Autodesk Inventor part; units mm, degrees
ref_plane "YZ Plane" through (0, 0, 0) normal (1, 0, 0) x (0, 1, 0)
ref_plane "XZ Plane" through (0, 0, 0) normal (0, 1, 0) x (-1, 0, 0)
ref_plane "XY Plane" through (0, 0, 0) normal (0, 0, 1) x (1, 0, 0)
sketch "sk_main" plane through (0, 0, 0) normal (1, 0, 0) x (0, 1, 0)
  line L0 (-8, 0) -> (30.5, 0)
  line L1 (0, -15.9) -> (0, 14.9)
  line L2 (25, -7.5) -> (0, -7.5)
  line L3 (0, -7.5) -> (0, 9)
  line L4 (25, -11.5) -> (-2.5, -11.5)
  line L5 (-2.5, -11.5) -> (-2.5, 10.5)
  line L6 (0, 10.5) -> (0, -11.5)
  line L7 (25, -7.5) -> (25, -11.5)
  line L8 (-2.5, 10.5) -> (0, 10.5)
  point P0 (0, 0)
  dimension "d5" = 2.5
  dimension "d35" = 25
  dimension "d37" = 4
  dimension "d38" = 18
  dimension "d58" = 10.5
extrude "ext_main_back" [suppressed]
extrude "ext_main_front" add sketch "sk_main" along normal mid plane 12.15 contours L5 L8 L1 L0 | L0 L1 L4 L5
sketch "sk_front" plane through (0, 0, 0) normal (0, 1, 0) x (-1, 0, 0)
  line L0 (0, -22.55) -> (0, 16.3)
  line L1 (12.1092, 0) -> (-12.1092, 0)
  circle A0 centre (0, 0) radius 3.4
  circle A1 centre (5.075, 0) radius 1
  circle A2 centre (-5.075, 0) radius 1
  circle A3 centre (0, 0) radius 8 construction
  circle A4 centre (0, -9) radius 8 construction
  circle A5 centre (0, -9) radius 1
  line L2 (8.6494, -4.5) -> (-8.6494, -4.5) construction
  line L3 (-6.075, 10.5) -> (-6.075, -11.5)
  line L4 (6.075, -11.5) -> (6.075, 10.5)
  line L5 (6.075, -11.5) -> (-6.075, -11.5)
  circle A6 centre (-5, 8.5) radius 1
  circle A7 centre (-5, 8.5) radius 2.25 construction
  line L6 (-5, 8.5) -> (5, 8.5) construction
  circle A8 centre (5, 8.5) radius 2.25 construction
  circle A9 centre (5, 8.5) radius 1
  line L7 (6.075, 10.5) -> (6.075, -11.5)
  line L8 (6.075, -11.5) -> (8.075, -11.5)
  line L9 (8.075, -11.5) -> (8.075, 10.5)
  line L10 (8.075, 10.5) -> (6.075, 10.5)
  line L11 (-6.075, -11.5) -> (-6.075, 10.5)
  line L12 (-6.075, 10.5) -> (-8.075, 10.5)
  line L13 (-8.075, 10.5) -> (-8.075, -11.5)
  line L14 (-8.075, -11.5) -> (-6.075, -11.5)
  point P0 (0, 8.5)
  dimension "d11" = 6.8
  dimension "d12" = 2
  dimension "d13" = 10.15
  dimension "d14" = 16
  dimension "d15" = 16
  dimension "d16" = 9
  dimension "d17" = 2
  dimension "d27" = 2
  dimension "d28" = 4.5
  dimension "d30" = 10
  dimension "d31" = 8.5
  dimension "d39" = 2
extrude "ext_front_tabs" add sketch "sk_front" against normal up to surface (2.5 mm away) contours L4 L1 L9 L8 | L14 L13 L1 L3 | L4 L10 L9 L1 | L1 L13 L12 L3
extrude "ext_cut_holesfront" cut sketch "sk_front" against normal through all contours A5 L0 | L0 A5 | A1 L1 | L1 A1 | A2 L1 | L1 A2 | A0 L1 L0 | L0 L1 A0 | L1 A0 L0 | L0 A0 L1 | A6 | A9
fillet "Fillet5" radius 2 4 edges at (-8.075, -1.25, -11.5) (8.075, -1.25, -11.5) (8.075, -1.25, 10.5) (-8.075, -1.25, 10.5)
sketch "Sketch7" plane through (8.075, 0, 8.5) normal (0, 1, 0) x (1, 0, 0)
  line L0 (0, 0) -> (0, 18)
  arc A0 (0, 18) -> (-2, 20) centre (-2, 18) ccw
  line L1 (-14.15, 20) -> (-2, 20)
  arc A1 (-14.15, 20) -> (-16.15, 18) centre (-14.15, 18) ccw
  line L2 (-16.15, 18) -> (-16.15, 0)
  circle A2 centre (-8.075, 8.5) radius 3.4
  circle A3 centre (-8.075, 8.5) radius 9
  line L3 (-11.033, 17) -> (-16.15, 17)
  line L4 (-5.117, 17) -> (0, 17)
  line L5 (-2, -2) -> (-14.15, -2)
  line L6 (-16.15, 17) -> (-16.15, 21)
  line L7 (-16.15, 21) -> (0, 21)
  line L8 (0, 21) -> (0, 17)
  dimension "d45" = 18
  dimension "d46" = 3
  dimension "d57" = 1
extrude "ext_backtab" add sketch "Sketch7" along normal blind 15 contours L4 A3 L3 L2 A1 L1 A0 L0
sketch "Sketch8" plane through (6.075, -2.5, -11.5) normal (0, 0, -1) x (-1, 0, 0)
  line L0 (12.15, 0) -> (0, 0)
  line L1 (0, 17.5) -> (12.15, 17.5)
  line L2 (6.075, 0) -> (6.075, 17.5)
  circle A0 centre (0.825, 8) radius 1.5
  circle A1 centre (11.325, 8) radius 1.5
  line L3 (0.825, 8) -> (11.325, 8) construction
  point P0 (6.075, 2.5)
  dimension "d49" = 3
  dimension "d50" = 10.5
  dimension "d56" = 8
extrude "ext_cut_mountholes" cut sketch "Sketch8" against normal up to next
fillet "Fillet6" radius 2.5 2 edges at (5.5165, 0, -8.5) (-5.5165, 0, -8.5)
extrude "ext_dowelfill" add sketch "sk_front" against normal blind 1.7 contours A5 L0 | L0 A5
equation "\"d12\" = screw_m2_bore_selfthreading"
equation "\"d17\" = screw_m2_bore_selfthreading"
equation "\"d27\" = screw_m2_bore_selfthreading"
equation "\"d28\" = screw_m2_head_maxsize"
equation "\"d49\" = screw_m3_bore_selfthreading"
properties part number "empty"
Geometry: final body of the model. Coordinates: model frame, mm. A direction names the side the tool comes from. Round coordinates to 2 decimals unless told otherwise and drop trailing zeros. Loops run counter-clockwise (first coordinate to the right, second up) from the corner with the lowest first, then second, coordinate; pieces in that order, holes last. Notation, with made-up numbers: (22.5, 12) -> (38.5, 12) arc R19 ccw to (38.5, 33) -> close; hole circle Ø8 at (43, 60.25). An arc over 180 degrees is marked (long way). One line per question, with ' | ' between items. Start each with the question number.
1. Contact query for flat-ended pins moving along their axis: pin 1 (1 mm diameter, centred on x = 4.5, y = 12, fed in from +Z); pin 2 (2.5 mm diameter, centred on x = -5, z = 8.5, fed in from +Y); pin 3 (1.2 mm diameter, centred on x = -5.075, z = 0, fed in from +Y); pin 4 (5 mm diameter, centred on x = 0, y = 6.5, fed in from +Z). Output: stop coordinate, or through.
2. Mould query, pull axis X, two halves, no side actions, for faces 1 (the face through (0, -1.7, -9)), 2 (the face through (-7.474, -1.268, 9.93)), 3 (the face through (-4.06, 4.59, -10.02)), 4 (the face through (5, 9, -8.5)). Classes: pulls with the +X half, pulls with the -X half, needs draft (parallel to the pull), parting line crosses it, or undercut.
3. Section B-B on x = -5.25. Output: boundary loops of the cut face in (y, z), and give its area (3 significant figures).
4. Set-up query: faces 5 (the face through (-5, 9, -8.5)), 6 (the face through (0.74, -1.23, -3.32)), 7 (the face through (0, 7, -9)). Return all of +Z, -Z, +X, -X, +Y, -Y with unobstructed straight access to the full face (end or side cutting, diameter ignored); none if empty.
5. Section D-D on y = 12.5. Output: boundary loops of the cut face in (x, z) (3 decimals), and give its area (4 significant figures).
6. Line query: line 1 along Z through (x, y) = (-5, -1.4); line 2 along Z through (x, y) = (0, -2.3); line 3 along X through (y, z) = (-0.6, 0) (3 decimals). Output: solid intervals per line, ascending. Write a range as [from, to].
7. Section C-C on z = 2. Output: boundary loops of the cut face in (x, y) (3 decimals), and give its area (3 significant figures).
8. Section A-A on x = 0. Output: boundary loops of the cut face in (y, z).
Returned:
1) pin 1: stops at z = -8.5 | pin 2: stops at y = 0 | pin 3: passes through | pin 4: stops at z = -8.65
2) face 1: undercut | face 2: pulls with the -X half | face 3: undercut | face 4: needs draft
3) outline: (-2.5, -11.5) -> (4, -11.5) -> (4, -8.5) -> (2.5, -8.5) arc R2.5 cw to (0.37, -7.31) -> (0, -7.31) -> (0, -0.98) -> (-2.5, -0.98) -> close; (-2.5, 0.98) -> (0, 0.98) -> (0, 7.53) -> (-2.5, 7.53) -> close; (-2.5, 9.47) -> (0, 9.47) -> (0, 10.5) -> (-2.5, 10.5) -> close; (7, -11.5) -> (15, -11.5) -> (15, -8.5) -> (7, -8.5) -> close | area: 82.4 mm2
4) face 5: +Z, +X, -X, +Y | face 6: +Y, -Y | face 7: +Z, +Y
5) outline: (-8.075, -9.5) arc R2 ccw to (-6.075, -11.5) -> (6.075, -11.5) arc R2 ccw to (8.075, -9.5) -> (8.075, -8.5) -> (2.958, -8.5) arc R9 cw to (-2.958, -8.5) -> (-8.075, -8.5) -> close | area: 44.75 mm2
6) line 1: z = [-11.5, -1], [1, 7.5], [9.5, 10.5] | line 2: z = [-11.5, -10], [-8, -3.4], [3.4, 10.5] | line 3: x = [-8.075, -6.075], [-4.075, -3.4], [3.4, 4.075], [6.075, 8.075]
7) outline: (-8.075, -2.5) -> (-2.75, -2.5) -> (-2.75, 0) -> (-8.075, 0) -> close; (2.75, -2.5) -> (8.075, -2.5) -> (8.075, 0) -> (2.75, 0) -> close | area: 26.6 mm2
8) outline: (-2.5, -11.5) -> (15, -11.5) -> (15, -9) -> (0, -9) -> (0, -3.4) -> (-2.5, -3.4) -> (-2.5, -8) -> (-1.7, -8) -> (-1.7, -10) -> (-2.5, -10) -> close; (-2.5, 3.4) -> (0, 3.4) -> (0, 10.5) -> (-2.5, 10.5) -> close
